Geometry check sheet. Reference: drawing and pictorial views, mm from the part's lowest x, y, z. Coordinates: 2 decimals unless noted, no trailing zeros. Write each loop counter-clockwise with the first axis right and the second up, starting at its lowest first coordinate (ties: lowest second). Pieces come first, ordered by that corner, then holes. Notation, with made-up numbers: (8.5, 49) -> (36.5, 49) arc R22 ccw to (36.5, 86) -> close; hole circle Ø3 at (54.5, 1). An arc over 180 degrees is marked (long way). Answer in a Markdown table with one row per item.
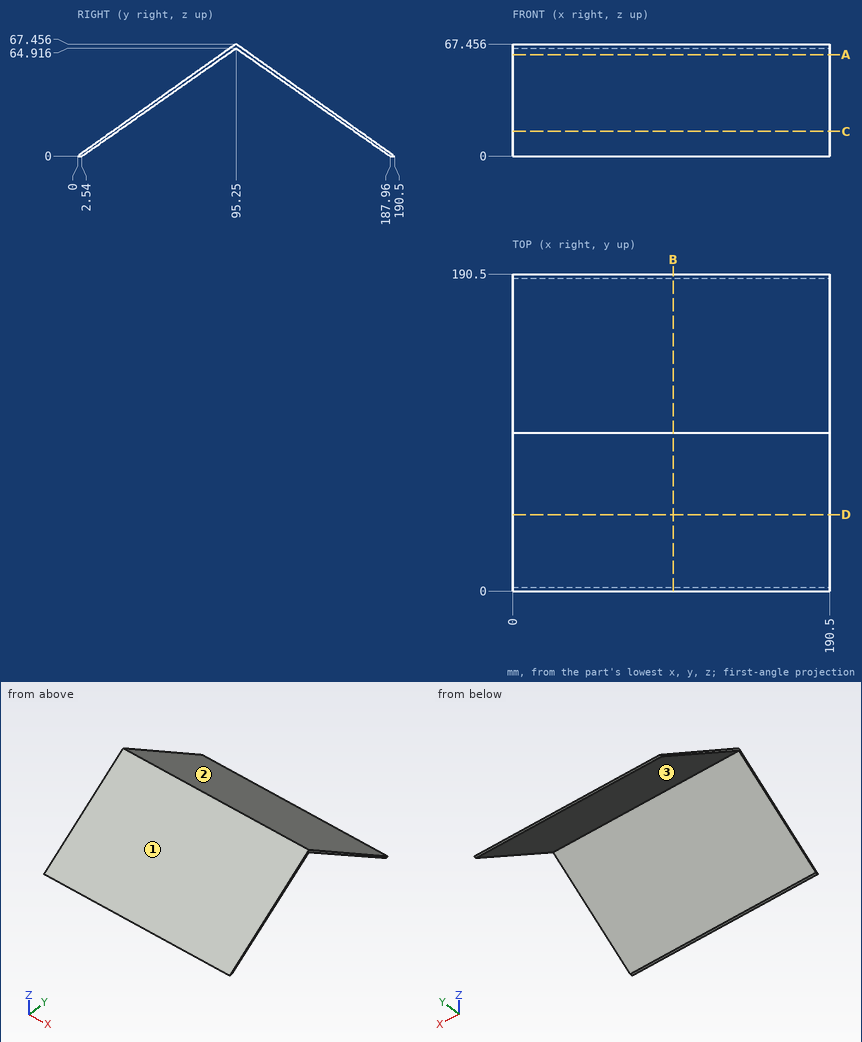
1. Section check C-C, the plane z = 15. Record the boundary of the cut face in (x, y), plus the area to 3 significant figures.
Geometry says:
| item | result |
|---|---|
| outline | (0, 21.18) -> (190.5, 21.18) -> (190.5, 23.96) -> (0, 23.96) -> close; (0, 166.54) -> (190.5, 166.54) -> (190.5, 169.32) -> (0, 169.32) -> close |
| area | 1,060 mm^2 |
2. Depth check by flat-ended pin: P1, Ø2, axis at x = 118.5, z = 35, coming from the +Y side; P2, Ø6, axis at x = 24, y = 39.5, coming from the +Z side; P3, Ø12, axis at x = 112.5, z = 59.5, coming from the -Y side. Enter the tip coordinate at first touch or a pass-through.
Geometry says:
| item | result |
|---|---|
| P1 | y = 142.49 |
| P2 | z = 30.1 |
| P3 | y = 75.54 |
3. Mould release check, pull along Y, two halves, no side actions. Record for the marked faces 1, 2 and 3: released by +Y, released by -Y, zero draft, split by the parting line, or undercut.
Geometry says:
| item | result |
|---|---|
| face 1 | released by -Y |
| face 2 | released by +Y |
| face 3 | undercut |
4. Section check A-A, the plane z = 61. Record the boundary of the cut face in (x, y).
Geometry says:
| item | result |
|---|---|
| outline | (0, 86.13) -> (190.5, 86.13) -> (190.5, 89.66) -> (0, 89.66) -> close; (0, 100.84) -> (190.5, 100.84) -> (190.5, 104.37) -> (0, 104.37) -> close |
5. Thickness scan on line 1 (Y direction, x = 181, z = 13.5); line 2 (Y direction, x = 159, z = 55); line 3 (Z direction, x = 14, y = 120.5) (1 decimal). Record the ranges inside material, lowest first. Write a range as from..to.
Geometry says:
| item | result |
|---|---|
| line 1 | 19.06..21.82, 168.68..171.44 |
| line 2 | 77.66..81.09, 109.41..112.84 |
| line 3 | 47.2..49.6 |
6. Section check D-D, the plane y = 46. Record the boundary of the cut face in (x, z).
Geometry says:
| item | result |
|---|---|
| outline | (0, 30.43) -> (190.5, 30.43) -> (190.5, 32.58) -> (0, 32.58) -> close |
7. Section check B-B, the plane x = 96.5. Record the boundary of the cut face in (y, z), plus the area to 3 significant figures.
Geometry says:
| item | result |
|---|---|
| outline | (0, 0) -> (2.54, 0) -> (95.25, 64.92) -> (187.96, 0) -> (190.5, 0) -> (95.25, 67.46) -> close |
| area | 407 mm^2 |
